```python
from build123d import *

# Parameters (mm, degrees)
SKETCH1_W                    = 68.58
SKETCH1_H                    = 43.18
BOSS_EXTRUDE1_DEPTH          = 2.54
SKETCH5_R                    = 2.54
BOSS_EXTRUDE2_DEPTH          = 2.54
SKETCH6_W                    = 68.58
SKETCH6_H                    = 43.18
BOSS_EXTRUDE3_DEPTH          = 12.7
SKETCH7_R                    = 1.4605
BOSS_EXTRUDE4_DEPTH          = 2.54
SKETCH8_W                    = 7.62
SKETCH8_H                    = 8.2856324
CUT_EXTRUDE1_DEPTH           = 83.46203005
SKETCH9_W                    = 16.129
SKETCH9_H                    = 8.382
CUT_EXTRUDE2_DEPTH           = 2.032
BOSS_EXTRUDE5_DEPTH          = 2.54
F_1_8_0_125_DIAMETER_HOLE1_D = 3.175


with BuildPart() as part:
    # Sketch1 → Boss-Extrude1 (new body)
    with BuildSketch(Plane(origin=(0, 0, 0), x_dir=(1, 0, 0), z_dir=(0, 1, 0))):
        with Locations((34.29, 21.59)):
            Rectangle(SKETCH1_W, SKETCH1_H)
    extrude(amount=BOSS_EXTRUDE1_DEPTH)

    # Sketch5 → Boss-Extrude2 (add)
    with BuildSketch(Plane(origin=(0, 2.54, 0), x_dir=(1, 0, 0), z_dir=(0, 1, 0))):
        with Locations(Location((5.715, 37.465, 0), (0, 0, 90))):
            Circle(SKETCH5_R)
        with Locations(Location((62.865, 37.465, 0), (0, 0, 90))):
            Circle(SKETCH5_R)
        with Locations(Location((5.715, 5.715, 0), (0, 0, 90))):
            Circle(SKETCH5_R)
        with Locations(Location((62.865, 5.715, 0), (0, 0, 90))):
            Circle(SKETCH5_R)
    extrude(amount=BOSS_EXTRUDE2_DEPTH)

    # Sketch6 → Boss-Extrude3 (add)
    with BuildSketch(Plane(origin=(0, 2.54, 0), x_dir=(1, 0, 0), z_dir=(0, 1, 0))):
        with Locations((34.29, 21.59)):
            Rectangle(SKETCH6_W, SKETCH6_H)
        Polygon((1.27, 42.171922196), (1.27, 1.27), (67.31, 1.27), (67.31, 42.229552983), align=None, mode=Mode.SUBTRACT)
    extrude(amount=BOSS_EXTRUDE3_DEPTH)

    # Sketch7 → Boss-Extrude4 (add)
    with BuildSketch(Plane(origin=(0, 5.08, 0), x_dir=(1, 0, 0), z_dir=(0, 1, 0))):
        with Locations(Location((5.715, 37.465, 0), (0, 0, 270))):
            Circle(SKETCH7_R)
        with Locations(Location((5.715, 5.715, 0), (0, 0, 270))):
            Circle(SKETCH7_R)
        with Locations(Location((62.865, 5.715, 0), (0, 0, 270))):
            Circle(SKETCH7_R)
        with Locations(Location((62.865, 37.465, 0), (0, 0, 270))):
            Circle(SKETCH7_R)
    extrude(amount=BOSS_EXTRUDE4_DEPTH)

    # Sketch8 → Cut-Extrude1 (cut, through all)
    with BuildSketch(Plane.XY):
        with Locations((12.446, 11.0971838)):
            Rectangle(SKETCH8_W, SKETCH8_H)
    extrude(amount=-CUT_EXTRUDE1_DEPTH, mode=Mode.SUBTRACT)

    # Sketch9 → Cut-Extrude2 (cut)
    with BuildSketch(Plane(origin=(68.58, 0, 0), x_dir=(0, 0, -1), z_dir=(1, 0, 0))):
        with Locations((16.4465, 11.049)):
            Rectangle(SKETCH9_W, SKETCH9_H)
    extrude(amount=-CUT_EXTRUDE2_DEPTH, mode=Mode.SUBTRACT)

    # Sketch10 → Boss-Extrude5 (add)
    with BuildSketch(Plane.XZ):
        with BuildLine():
            Line((0, 3.175), (0, 0))
            Line((0, 0), (6.35, 0))
            Line((6.35, 0), (6.35, 3.175))
            ThreePointArc((6.35, 3.175), (3.175, 6.35), (0, 3.175))
        make_face()
        with BuildLine():
            Line((6.35, -46.355), (6.35, -43.18))
            Line((6.35, -43.18), (0, -43.18))
            Line((0, -43.18), (0, -46.355))
            ThreePointArc((0, -46.355), (3.175, -49.53), (6.35, -46.355))
        make_face()
        with BuildLine():
            Line((68.58, -46.355), (68.58, -43.18))
            Line((68.58, -43.18), (62.23, -43.18))
            Line((62.23, -43.18), (62.23, -46.355))
            ThreePointArc((62.23, -46.355), (65.405, -49.53), (68.58, -46.355))
        make_face()
        with BuildLine():
            Line((62.23, 3.175), (62.23, 0))
            Line((62.23, 0), (68.58, 0))
            Line((68.58, 0), (68.58, 3.175))
            ThreePointArc((68.58, 3.175), (65.405, 6.35), (62.23, 3.175))
        make_face()
    extrude(amount=-BOSS_EXTRUDE5_DEPTH)

    # 1/8 (0.125) Diameter Hole1 (through all)
    with Locations(Plane(origin=(0, 2.54, 0), x_dir=(1, 0, 0), z_dir=(0, 1, 0))):
        with Locations((65.405, 46.355), (3.175, 46.355), (3.175, -3.175), (65.405, -3.175)):
            Hole(F_1_8_0_125_DIAMETER_HOLE1_D / 2)


solid = part.part
```
The model under review builds one solid part; all positions refer to its coordinate system, in mm. A direction names the side the tool comes from. Give positions to 0.01 mm unless a question says otherwise; leave off trailing zeros. Write each loop counter-clockwise with the first axis right and the second up, starting at its lowest first coordinate (ties: lowest second). Pieces come first, ordered by that corner, then holes. Notation, with made-up numbers: (-28.5, -31) -> (-5.5, -31) arc R16 ccw to (-5.5, -11) -> close; hole circle Ø3 at (-34, 22). An arc over 180 degrees is marked (long way). Answer in a Markdown table with one row per item.
1) Tool access review of faces 1 (the flat face through (6.35, 1, -45)), 2 (the flat face through (62.23, 1, 2)), 3 (the flat face through (1.27, 9, -22)), 4 (the flat face through (2, 2.54, -45)), 5 (the flat face through (3, 2.54, 1)): name each direction out of +Z, -Z, +X, -X, +Y, -Y from which nothing blocks a thin tool from reaching the whole face with its end or side.
Worked answers:
| item | result |
|---|---|
| face 1 | -Z, +Y, -Y |
| face 2 | +Z, +Y, -Y |
| face 3 | +Y |
| face 4 | -Z, +X, -X, +Y |
| face 5 | +Z, +X, -X, +Y |
2) Clearance check with flat-ended pins moving along their axes: P1, Ø1, axis at x = 46.5, y = 3.5, coming from the -Z side; P2, Ø5, axis at x = 65.5, z = -47, coming from the +Y side; P3, Ø12, axis at x = 12, z = -39, coming from the -Y side; P4, Ø4, axis at x = 5.5, z = -4.5, coming from the +Y side. State where each tip first meets the part, or that it passes through.
Worked answers:
| item | result |
|---|---|
| P1 | z = -43.18 |
| P2 | y = 2.54 |
| P3 | y = 0 |
| P4 | y = 7.62 |
3) Add section A-A on y = 3.75. State the section outline as (x, z) points (3 decimals).
Worked answers:
| item | result |
|---|---|
| outline | (0, -43.18) -> (68.58, -43.18) -> (68.58, 0) -> (0, 0) -> close; circle Ø5.08 at (5.715, -37.465); circle Ø5.08 at (5.715, -5.715); circle Ø5.08 at (62.865, -37.465); circle Ø5.08 at (62.865, -5.715); hole (1.27, -42.172) -> (67.31, -42.23) -> (67.31, -1.27) -> (1.27, -1.27) -> close |
4) Mouldability with a two-part tool opening along Z and no side actions: class faces 6 (the cylindrical face through (65.47, 1.25, 6.35)), 7 (the flat face through (46, 15.24, -1)), 8 (the cylindrical face through (61.57, 6.33, -5.04)) as +Z half, -Z half, draft (parallel to the pull), parting line (faces both ways), or undercut.
Worked answers:
| item | result |
|---|---|
| face 6 | +Z half |
| face 7 | draft |
| face 8 | undercut |
5) For L1, parallel to X at y = 2, z = -44; L2, parallel to X at y = 4.75, z = -33; L3, parallel to Z at x = 64, y = 2.25, list the stretches that pass through material, from the lowest coordinate up. Write a range as [from, to].
Worked answers:
| item | result |
|---|---|
| L1 | [0, 6.35], [62.23, 68.58] |
| L2 | [0, 1.27], [67.31, 68.58] |
| L3 | [-49.2, -47.09], [-45.62, 2.44], [3.91, 6.02] |
6) Add section B-B on z = -16.5. State the section outline as (x, y) points, plus the area to 3 significant figures.
Worked answers:
| item | result |
|---|---|
| outline | (0, 0) -> (68.58, 0) -> (68.58, 6.86) -> (67.31, 6.86) -> (67.31, 2.54) -> (1.27, 2.54) -> (1.27, 15.24) -> (0, 15.24) -> close |
| area | 196 mm² |
7) Add section C-C on y = 9.75. State the section outline as (x, z) points (3 decimals).
Worked answers:
| item | result |
|---|---|
| outline | (0, -43.18) -> (8.636, -43.18) -> (8.636, -42.178) -> (1.27, -42.172) -> (1.27, -1.27) -> (8.636, -1.27) -> (8.636, 0) -> (0, 0) -> close; (16.256, -43.18) -> (68.58, -43.18) -> (68.58, -24.511) -> (67.31, -24.511) -> (67.31, -42.23) -> (16.256, -42.185) -> close; (16.256, -1.27) -> (67.31, -1.27) -> (67.31, -8.382) -> (68.58, -8.382) -> (68.58, 0) -> (16.256, 0) -> close |
8) Add section D-D on x = 41. State the section outline as (y, z) points, plus the area to 3 significant figures.
Worked answers:
| item | result |
|---|---|
| outline | (0, -43.18) -> (15.24, -43.18) -> (15.24, -42.21) -> (2.54, -42.21) -> (2.54, -1.27) -> (15.24, -1.27) -> (15.24, 0) -> (0, 0) -> close |
| area | 138 mm² |
